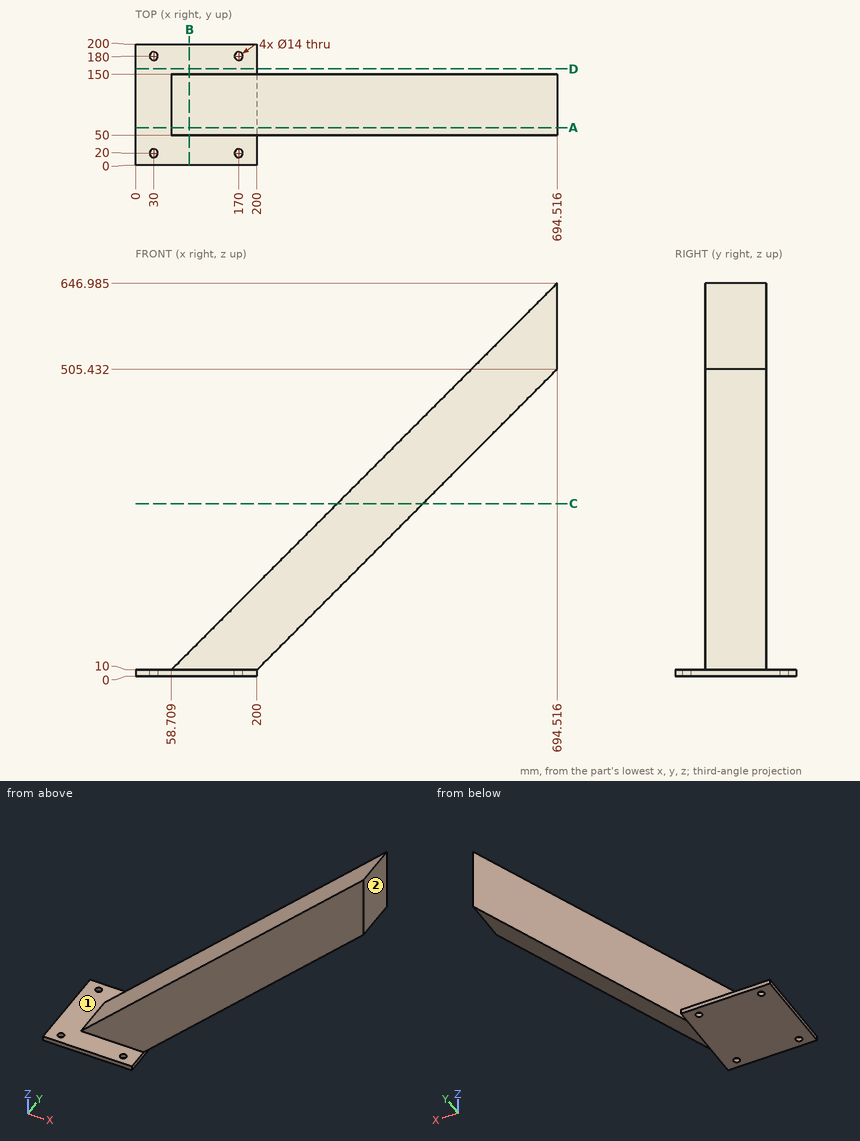
Print and shaded views of the part. All mm, measured from the part's lowest x, y and z. A direction names the side the tool comes from. Coordinates: 2 decimals unless noted, no trailing zeros. Order: outer loops, then holes, each group sorted by start corner. A loop starts at its lowest first (then second) coordinate and runs counter-clockwise, first axis right, second up. Notation, with made-up numbers: (83.5, 42.25) - (106.5, 42.25) arc R26 cw to (106.5, 67.25) - close; hole circle Ø9 at (-17, 43). An arc over 180 degrees is marked (long way). Put each result on its own line as item: value.
1. Saw through at C-C (z = 284). Write the cut outline in (x, y).
Answer sheet:
outline: (332.2, 50) - (473.49, 50) - (473.49, 150) - (332.2, 150) - close
2. Tool access for the marked faces 1 and 2: list every direction of +Z, -Z, +X, -X, +Y, -Y with a clear straight run to the whole face (end or side of a thin tool).
Answer sheet:
face 1: +Z, -X
face 2: +Z, -Z, +X, +Y, -Y
3. Probe line 1 along Y through (x, z) = (170, 3); line 2 along X through (y, z) = (180, 6); line 3 along Z through (x, y) = (143, 187.5). List the from-to ranges inside material, lowest first. Write a range as [from, to].
Answer sheet:
line 1: y = [0, 13], [27, 173], [187, 200]
line 2: x = [0, 23], [37, 163], [177, 200]
line 3: z = [0, 10]
4. Drop flat-ended pins along their axis: P1, Ø22.5, axis at x = 170, y = 180, coming from the +Z side; P2, Ø11, axis at y = 100, z = 5.5, coming from the +X side; P3, Ø12, axis at y = 118.5, z = 122.5, coming from the +X side; P4, Ø11, axis at x = 170, y = 20, coming from the -Z side. Give the stop position or say it passes through.
Answer sheet:
P1: stops at z = 10
P2: stops at x = 201
P3: stops at x = 318.28
P4: passes through
5. Saw through at B-B (x = 88.5). Write the cut outline in (y, z).
Answer sheet:
outline: (0, 0) - (200, 0) - (200, 10) - (150, 10) - (150, 39.85) - (50, 39.85) - (50, 10) - (0, 10) - close
6. Saw through at D-D (y = 159). Write the cut outline in (x, z).
Answer sheet:
outline: (0, 0) - (200, 0) - (200, 10) - (0, 10) - close
7. Saw through at A-A (y = 62). Write the cut outline in (x, z) (1 decimal), and give its area (3 significant figures).
Answer sheet:
outline: (0, 0) - (200, 0) - (200, 10) - (694.5, 505.4) - (694.5, 647) - (58.7, 10) - (0, 10) - close
area: 82,000 mm^2
